Verification items for the finished model (mm, model axes). Face numbers are marked on the shaded views. A direction names the side the tool comes from. Give positions to 0.01 mm unless a question says otherwise; leave off trailing zeros. Loops run counter-clockwise (first coordinate to the right, second up) from the corner with the lowest first, then second, coordinate; pieces in that order, holes last. Notation, with made-up numbers: M -24,-15 L -9,-15 A23 ccw -9,17 Z; hole C -38,-5 d11. An arc over 180 degrees is marked long. Use CSV: the item, a comma, the result in double quotes.
from build123d import *
from build123d import SkipClean  # not in build123d's __all__

# Parameters (mm, degrees)
F0_R     = 6.35
F1_DEPTH = 12.7
F2_R     = 6.35
F3_DEPTH = 12.7
F4_R     = 6.35
F5_DEPTH = 12.7


# Not quite as in the source:
# - after a boolean that leaves OpenCascade's solid faulty, fix() repairs it


with BuildPart() as f1:
    # F0 (on Front) → F1 (new body)
    with BuildSketch(Plane.XZ):
        with BuildLine():
            ThreePointArc((-12.7, 0), (0, -12.7), (12.7, 0))
            ThreePointArc((12.7, 0), (0, 12.7), (-12.7, 0))
        make_face()
        Circle(F0_R, mode=Mode.SUBTRACT)
        with BuildLine():
            Line((12.7, -63.5), (12.7, 0))
            ThreePointArc((12.7, 0), (0, -12.7), (-12.7, 0))
            Line((-12.7, 0), (-12.7, -63.5))
            ThreePointArc((-12.7, -63.5), (0, -50.8), (12.7, -63.5))
        make_face()
        with BuildLine():
            ThreePointArc((-12.7, -63.5), (0, -76.2), (12.7, -63.5))
            ThreePointArc((12.7, -63.5), (0, -50.8), (-12.7, -63.5))
        make_face()
        with Locations((0, -63.5)):
            Circle(F0_R, mode=Mode.SUBTRACT)
    extrude(amount=F1_DEPTH)

    # F2 (on face) → F3 (join)
    with BuildSketch(Plane(origin=(0, 0, 0), x_dir=(-1, 0, 0), z_dir=(0, 1, 0))):
        with BuildLine():
            ThreePointArc((3.3866666667, -12.2401180096), (10.1069448071, -7.6902318994), (12.7, 0))
            ThreePointArc((12.7, 0), (7.6902318994, 10.1069448071), (-3.3866666667, 12.2401180096))
            ThreePointArc((-3.3866666667, 12.2401180096), (-12.2401180096, -3.3866666667), (3.3866666667, -12.2401180096))
        make_face()
        Circle(F2_R, mode=Mode.SUBTRACT)
        with BuildLine():
            ThreePointArc((3.3866666667, -12.2401180096), (-12.2401180096, -3.3866666667), (-3.3866666667, 12.2401180096))
            Line((-3.3866666667, 12.2401180096), (-76.8273747243, -8.0798819904))
            ThreePointArc((-76.8273747243, -8.0798819904), (-65.7504761582, -10.2130551929), (-60.7407080576, -20.32))
            ThreePointArc((-60.7407080576, -20.32), (-63.3337632505, -28.0102318994), (-70.0540413909, -32.5601180096))
            Line((-70.0540413909, -32.5601180096), (3.3866666667, -12.2401180096))
        make_face()
        with BuildLine():
            ThreePointArc((-60.7407080576, -20.32), (-65.7504761582, -10.2130551929), (-76.8273747243, -8.0798819904))
            ThreePointArc((-76.8273747243, -8.0798819904), (-85.6808260672, -23.7066666667), (-70.0540413909, -32.5601180096))
            ThreePointArc((-70.0540413909, -32.5601180096), (-63.3337632505, -28.0102318994), (-60.7407080576, -20.32))
        make_face()
        with Locations((-73.4407080576, -20.32)):
            Circle(F2_R, mode=Mode.SUBTRACT)
    with SkipClean():  # cleaning this boolean's faces spoils the solid; the shape is the same uncleaned
        extrude(amount=F3_DEPTH)

    # F4 (on face) → F5 (join)
    with BuildSketch(Plane.XZ):
        with BuildLine():
            ThreePointArc((62.4421854295, -26.67), (76.7277099304, -32.5872579939), (86.1407080576, -20.32))
            ThreePointArc((86.1407080576, -20.32), (85.7079660515, -17.0329981272), (84.4392306857, -13.97))
            ThreePointArc((84.4392306857, -13.97), (67.0907080576, -9.3214773719), (62.4421854295, -26.67))
        make_face()
        with Locations((73.4407080576, -20.32)):
            Circle(F4_R, mode=Mode.SUBTRACT)
        with BuildLine():
            ThreePointArc((84.4392306857, -13.97), (85.7079660515, -17.0329981272), (86.1407080576, -20.32))
            ThreePointArc((86.1407080576, -20.32), (76.7277099304, -32.5872579939), (62.4421854295, -26.67))
            Line((62.4421854295, -26.67), (100.5421854295, -92.6611357684))
            ThreePointArc((100.5421854295, -92.6611357684), (105.1907080576, -75.3126131403), (122.5392306857, -79.9611357684))
            Line((122.5392306857, -79.9611357684), (84.4392306857, -13.97))
        make_face()
        with BuildLine():
            ThreePointArc((124.2407080576, -86.3111357684), (123.8079660515, -83.0241338956), (122.5392306857, -79.9611357684))
            ThreePointArc((122.5392306857, -79.9611357684), (105.1907080576, -75.3126131403), (100.5421854295, -92.6611357684))
            ThreePointArc((100.5421854295, -92.6611357684), (114.8277099304, -98.5783937622), (124.2407080576, -86.3111357684))
        make_face()
        with Locations((111.5407080576, -86.3111357684)):
            Circle(F4_R, mode=Mode.SUBTRACT)
    extrude(amount=F5_DEPTH)

    add(f1.part.fix(), mode=Mode.REPLACE)


solid = f1.part
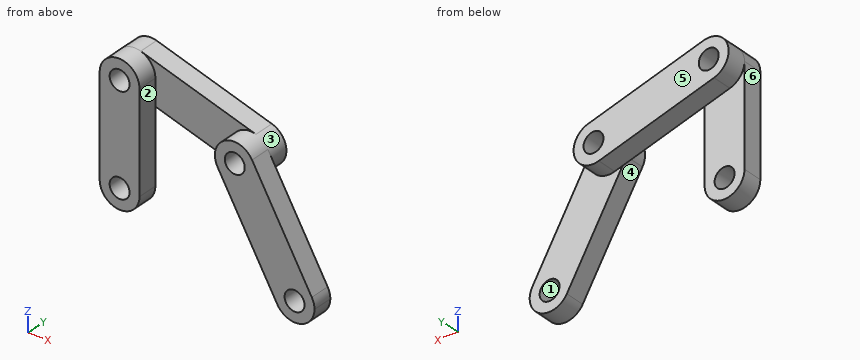
(1) Depth check by flat-ended pin: pin 1 Ø10 at (y, z) = (-8.5, -36) entering from +X (3 decimals); pin 2 Ø7.5 at (x, z) = (-5, -36.5) entering from +Y; pin 3 Ø21.5 at (x, z) = (33, -19.5) entering from -Y. Enter the tip coordinate at first touch or a pass-through.
Calculated:
pin 1,"stops at x = 100.045"
pin 2,"stops at y = 0"
pin 3,"stops at y = 0"
(2) Section check A-A on z = -90. Record the cut outline in (x, y).
Calculated:
outline,"M 99.01,-12.7 L 106.37,-12.7 L 106.37,0 L 99.01,0 Z; M 116.71,-12.7 L 123.69,-12.7 L 123.69,0 L 116.71,0 Z"
(3) Tool access check on the marked faces 1, 2 and 3. Record the directions out of +Z, -Z, +X, -X, +Y, -Y that give a thin tool (end or side, any length) a straight path to the whole face; none if there is none.
Calculated:
face 1,"+Y, -Y"
face 2,"+Z, -Z, -Y"
face 3,"none"
(4) Mould release check, pull along X, two halves, no side actions. Record for the marked faces 4, 5 and 6: released by +X, released by -X, zero draft, split by the parting line, or undercut.
Calculated:
face 4,"undercut"
face 5,"zero draft"
face 6,"released by -X"
(5) Scan line: L1, parallel to Y at x = 79.5, z = -45.5. Record every from-to range of solid material in increasing order. Write a range as from..to.
Calculated:
L1,"y = -12.7..0"
